Can you work these out from the drawing? Everything is in mm from the part's minimum corner. A direction names the side the tool comes from. Round coordinates to 2 decimals unless told otherwise and drop trailing zeros. Order: outer loops, then holes, each group sorted by start corner. A loop starts at its lowest first (then second) coordinate and runs counter-clockwise, first axis right, second up. Notation, with made-up numbers: M 19,21.5 L 47,21.5 A21 cw 47,55.5 Z; hole C 46.25,20 d5. An arc over 180 degrees is marked long. Answer as a JSON object with one key per item and string values. Group by question number.
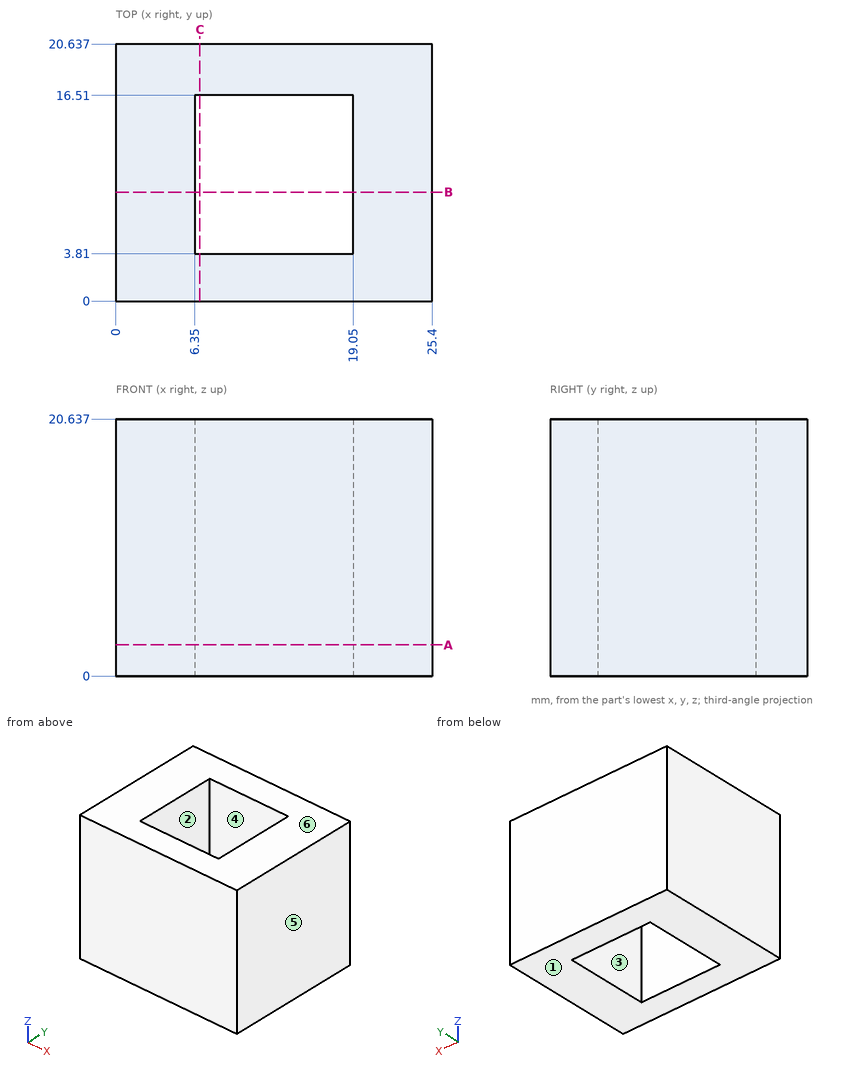
Item 1: If we mould it in two halves opening along X, with no side actions, what happens to the marked faces 3, 4, 5 and 6? For each: +X half, -X half, draft (parallel to the pull), parting line (faces both ways), or undercut.
Item 2: Suppose I cut it at B-B, the plane y = 8.75. Write out the boundary of the cut face in (x, z), and give its area (3 significant figures).
Item 3: On a 3-axis mill with a long thin cutter (end or side, diameter ignored), from which of +Z, -Z, +X, -X, +Y, -Y can I reach the whole of each face in a straight line? I mean the marked faces 1 and 2. Say none if no direction works.
Item 4: Suppose I cut it at C-C, the plane x = 6.75. Write out the boundary of the cut face in (y, z).
Item 5: Suppose I cut it at A-A, the plane z = 2.5. Write out the boundary of the cut face in (x, y), and give its area (3 significant figures).
Item 6: I need wall thicknesses on line 1 (X direction, y = 9.5, z = 18.75); line 2 (Y direction, x = 14, z = 12.25). Which ranges of each line are inside material? Lowest first, please.
Item 7: I'm going to push a flat-ended pin straight in: pin 1 Ø12 at (x, z) = (11, 10.5) entering from -Y. Where does the tip first touch, or does it pass through?
Computed:
{
 "1": {"face 3": "undercut", "face 4": "undercut", "face 5": "+X half", "face 6": "draft"},
 "2": {"outline": "M 0,0 L 6.35,0 L 6.35,20.64 L 0,20.64 Z; M 19.05,0 L 25.4,0 L 25.4,20.64 L 19.05,20.64 Z", "area": "262 mm^2"},
 "3": {"face 1": "-Z, +X, -X, +Y, -Y", "face 2": "+Z, -Z"},
 "4": {"outline": "M 0,0 L 3.81,0 L 3.81,20.64 L 0,20.64 Z; M 16.51,0 L 20.64,0 L 20.64,20.64 L 16.51,20.64 Z"},
 "5": {"outline": "M 0,0 L 25.4,0 L 25.4,20.64 L 0,20.64 Z; hole M 6.35,3.81 L 19.05,3.81 L 19.05,16.51 L 6.35,16.51 Z", "area": "363 mm^2"},
 "6": {"line 1": "x = 0 to 6.35, 19.05 to 25.4", "line 2": "y = 0 to 3.81, 16.51 to 20.64"},
 "7": {"pin 1": "stops at y = 0"}
}
